```python
from build123d import *

# Parameters (mm, degrees)
F1_DEPTH = 2


with BuildPart() as f1:
    # F0 (on Top) → F1 (new body)
    with BuildSketch(Plane.XY):
        Polygon((-20, -7.397476), (0, -7.397476), (20, -7.397476), (20, 32.602524), (0, 32.602524), (-20, 32.602524), align=None)
        Polygon((6.15, 26.7), (9.5, 25.7), (14, 20), (13.3, 4.2), (9.6, 0.5), (0, 0), (-9.6, 0.5), (-13.3, 4.2), (-14, 20), (-9.5, 25.7), (-6.15, 26.7), (0, 27.5), align=None, mode=Mode.SUBTRACT)
    extrude(amount=F1_DEPTH)


solid = f1.part
```
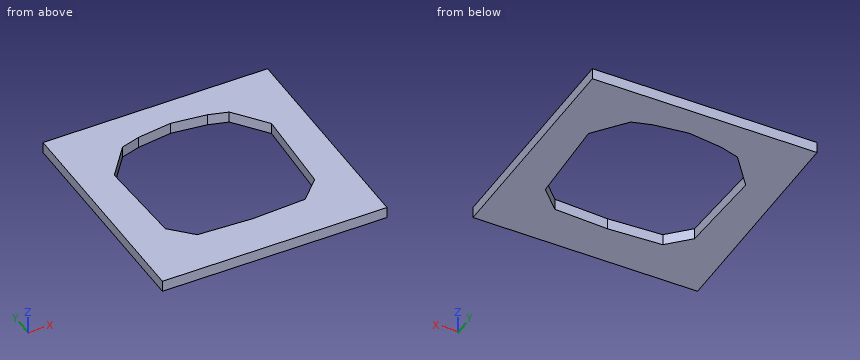
Here's how the part is built. I have some questions about the finished solid (model axes, mm). Coordinates: 2 decimals unless noted, no trailing zeros. Order: outer loops, then holes, each group sorted by start corner. A loop starts at its lowest first (then second) coordinate and runs counter-clockwise, first axis right, second up.
Item 1: If we section it at A-A, the plane y = 2.5: List the corners of the cut face in (x, z) for me.
Response values:
outline: (-20, 0) - (-11.6, 0) - (-11.6, 2) - (-20, 2) - close; (11.6, 0) - (20, 0) - (20, 2) - (11.6, 2) - close
Item 2: If we section it at C-C, the plane z = 0.75: List the corners of the cut face in (x, y) for me, then the cut area to 3 significant figures.
Response values:
outline: (-20, -7.4) - (20, -7.4) - (20, 32.6) - (-20, 32.6) - close; hole (-14, 20) - (-13.3, 4.2) - (-9.6, 0.5) - (0, 0) - (9.6, 0.5) - (13.3, 4.2) - (14, 20) - (9.5, 25.7) - (6.15, 26.7) - (0, 27.5) - (-6.15, 26.7) - (-9.5, 25.7) - close
area: 925 mm2
Item 3: If we section it at B-B, the plane x = -8.5: List the corners of the cut face in (y, z) for me, then the cut area to 3 significant figures.
Response values:
outline: (-7.4, 0) - (0.44, 0) - (0.44, 2) - (-7.4, 2) - close; (26, 0) - (32.6, 0) - (32.6, 2) - (26, 2) - close
area: 28.9 mm2
Item 4: I need wall thicknesses on probe 1 along Y at (x, z) = (9.5, 0.7); probe 2 along X at (y, z) = (12.5, 1.4); probe 3 along Y at (x, z) = (-8.5, 0.55). Which ranges of each line are inside material? Lowest first, please.
Response values:
probe 1: y = -7.4 to 0.49, 25.7 to 32.6
probe 2: x = -20 to -13.67, 13.67 to 20
probe 3: y = -7.4 to 0.44, 26 to 32.6
